from build123d import *

# Parameters (mm, degrees)
SKETCH_R        = 12
SKETCH_R_2      = 8.5
PAD_DEPTH       = 2
SKETCH001_R     = 3
SKETCH001_R_2   = 8.5
PAD001_DEPTH    = 5
SKETCH002_R     = 8.5
PAD002_DEPTH    = 3
SKETCH003_R     = 6.9
PAD003_DEPTH    = 2
PAD004_DEPTH    = 4.5
SKETCH005_R     = 2
PAD005_DEPTH    = 4
FILLET_R        = 3
CHAMFER_SIZE    = 0.4
CHAMFER001_SIZE = 0.4
SKETCH006_R     = 3
POCKET_DEPTH    = 4.001


with BuildPart() as part:
    # Sketch → Pad (new body)
    with BuildSketch(Plane.XY):
        Circle(SKETCH_R)
        Circle(SKETCH_R_2, mode=Mode.SUBTRACT)
    extrude(amount=PAD_DEPTH)

    # Sketch001 (on Face4 of Pad) → Pad001 (join)
    with BuildSketch(Plane.XY.offset(2)):
        with BuildLine():
            ThreePointArc((-1.128054, -11.946861), (12.25, -21.217622), (10.910313, -4.996507))
            ThreePointArc((10.910313, -4.996507), (-6, 10.392305), (-1.128054, -11.946861))
        make_face()
        with Locations((7.75, -13.423394)):
            Circle(SKETCH001_R, mode=Mode.SUBTRACT)
        Circle(SKETCH001_R_2, mode=Mode.SUBTRACT)
    extrude(amount=-PAD001_DEPTH)

    # Sketch002 (on Face6 of Pad001) → Pad002 (join)
    with BuildSketch(Plane(origin=(0, 0, -3), x_dir=(1, 0, 0), z_dir=(0, 0, -1))):
        Circle(SKETCH002_R)
    extrude(amount=-PAD002_DEPTH)

    # Sketch003 (on Face11 of Pad002) → Pad003 (join)
    with BuildSketch(Plane.XY):
        Circle(SKETCH003_R)
    extrude(amount=PAD003_DEPTH)

    # Sketch004 (on Face7 of Pad003) → Pad004 (join)
    with BuildSketch(Plane.XY.offset(2)):
        with BuildLine():
            Line((-0.800254, -10.613919), (5.90795, -22.232869))
            ThreePointArc((-0.800254, -10.613919), (-0.044229, -17.923394), (5.90795, -22.232869))
        make_face()
        with BuildLine():
            Line((16.300254, -16.232869), (9.59205, -4.613919))
            ThreePointArc((16.300254, -16.232869), (15.544229, -8.923394), (9.59205, -4.613919))
        make_face()
    extrude(amount=PAD004_DEPTH)

    # Sketch005 (on Face19 of Pad004) → Pad005 (join)
    with BuildSketch(Plane.XY.offset(-3)):
        with BuildLine():
            Line((-39.5, 16), (17.5, 16))
            Line((17.5, 16), (24.5, 16))
            Line((24.5, 16), (30.5, 16))
            Line((30.5, 16), (30.5, -16))
            Line((24.5, -16), (30.5, -16))
            Line((17.5, -16), (24.5, -16))
            Line((17.5, -16), (16.373288, -16))
            ThreePointArc((-0.873288, -16), (7.75, -22.423394), (16.373288, -16))
            Line((-0.873288, -16), (-39.5, -16))
            Line((-39.5, -16), (-39.5, 16))
        make_face()
        with Locations((-35.5, 5)):
            Circle(SKETCH005_R, mode=Mode.SUBTRACT)
        with Locations((-35.5, -5)):
            Circle(SKETCH005_R, mode=Mode.SUBTRACT)
        with Locations((13.5, 5)):
            Circle(SKETCH005_R, mode=Mode.SUBTRACT)
        with Locations((13.5, -5)):
            Circle(SKETCH005_R, mode=Mode.SUBTRACT)
        with Locations((-35.5, 12)):
            Circle(SKETCH005_R, mode=Mode.SUBTRACT)
        with Locations((-35.5, -12)):
            Circle(SKETCH005_R, mode=Mode.SUBTRACT)
        with Locations((20.5, 12)):
            Circle(SKETCH005_R, mode=Mode.SUBTRACT)
        with Locations((20.5, -12)):
            Circle(SKETCH005_R, mode=Mode.SUBTRACT)
        with Locations((26.5, -12)):
            Circle(SKETCH005_R, mode=Mode.SUBTRACT)
        with Locations((26.5, 12)):
            Circle(SKETCH005_R, mode=Mode.SUBTRACT)
    extrude(amount=-PAD005_DEPTH)

    # Fillet
    fillet_edges = [part.edges().sort_by_distance(p)[0] for p in [
        (-39.5, -16, -5),
        (30.5, -16, -5),
        (30.5, 16, -5),
        (-39.5, 16, -5),
    ]]
    fillet(fillet_edges, radius=FILLET_R)

    # Chamfer
    chamfer_edges = [part.edges().sort_by_distance(p)[0] for p in [
        (-6.9, 0, 2),
    ]]
    chamfer(chamfer_edges, length=CHAMFER_SIZE)

    # Chamfer001
    chamfer001_edges = [part.edges().sort_by_distance(p)[0] for p in [
        (-8.5, 0, 2),
    ]]
    chamfer(chamfer001_edges, length=CHAMFER001_SIZE)

    # Sketch006 (on Face23 of Chamfer001) → Pocket (cut, through all)
    with BuildSketch(Plane.XY.offset(-3)):
        with Locations((7.75, -13.423394)):
            Circle(SKETCH006_R)
    extrude(amount=-POCKET_DEPTH, mode=Mode.SUBTRACT)


solid = part.part
The listing builds one solid part. Answer for the finished solid, in the listing's coordinates (mm). A direction names the side the tool comes from. Coordinates: 2 decimals unless noted, no trailing zeros. Order: outer loops, then holes, each group sorted by start corner. A loop starts at its lowest first (then second) coordinate and runs counter-clockwise, first axis right, second up.
Q1. A cutting plane is placed at D-D, the plane y = 11. Write down the section's boundary in (x, z).
Q2. A cutting plane is placed at C-C, the plane z = -4.5. State how many separate pieces and enclosed holes the cut face has, and give its area (3 significant figures).
Q3. Given P1, Ø4, axis at y = 1, z = 5, coming from the -X side; P2, Ø3, axis at x = 21, z = -5, coming from the -Y side; P3, Ø8, axis at x = 5, y = -11.5, coming from the +Z side; P4, Ø8, axis at x = -4, z = 0.5, coming from the -Y side, each flat-ended and moving along its own axis, determine where each tip first touches the part or whether it passes through.
Q4. A cutting plane is placed at A-A, the plane x = 26.5. Write down the section's boundary in (y, z), and give its area (3 significant figures).
Q5. For a pull along Y with two mould halves and no side action, classify faces 4 (the face through (-18, -16, -5)), 5 (the face through (0, 0, 2)), 6 (the face through (-5, 16, -5)), 7 (the face through (-1, -7, 0)) as pulls with the +Y half, pulls with the -Y half, needs draft (parallel to the pull), parting line crosses it, or undercut.
Q6. A cutting plane is placed at B-B, the plane x = -35.5. Write down the section's boundary in (y, z).
Q7. Which of the six approach directions +Z, -Z, +X, -X, +Y, -Y give full straight-line access (tool end or side, diameter ignored) to faces 1 (the face through (11.9, -6.2, -5)), 2 (the face through (22, -16, -5)), 3 (the face through (-33.653, -5.766, -4.972))?
Q8. Consider line 1 (Y direction, x = -35.5, z = -5.95); line 2 (Y direction, x = 25.5, z = -3.5); line 3 (Y direction, x = 26, z = -4.75). Determine where each line is inside the solid, lowest interval first.
Answers follow:
1. outline: (-39.5, -7) - (-37.23, -7) - (-37.23, -3) - (-39.5, -3) - close; (-33.77, -7) - (18.77, -7) - (18.77, -3) - (4.8, -3) - (4.8, 2) - (-4.8, 2) - (-4.8, -3) - (-33.77, -3) - close; (22.23, -7) - (24.77, -7) - (24.77, -3) - (22.23, -3) - close; (28.23, -7) - (30.5, -7) - (30.5, -3) - (28.23, -3) - close
2. separate pieces: 1
2. enclosed holes: 11
2. area: 2,160 mm2
3. P1: passes through
3. P2: stops at y = -16
3. P3: stops at z = 2
3. P4: stops at y = -18
4. outline: (-16, -7) - (-14, -7) - (-14, -3) - (-16, -3) - close; (-10, -7) - (10, -7) - (10, -3) - (-10, -3) - close; (14, -7) - (16, -7) - (16, -3) - (14, -3) - close
4. area: 96.0 mm2
5. face 4: pulls with the -Y half
5. face 5: needs draft
5. face 6: pulls with the +Y half
5. face 7: undercut
6. outline: (-16, -7) - (-14, -7) - (-14, -3) - (-16, -3) - close; (-10, -7) - (-7, -7) - (-7, -3) - (-10, -3) - close; (-3, -7) - (3, -7) - (3, -3) - (-3, -3) - close; (7, -7) - (10, -7) - (10, -3) - (7, -3) - close; (14, -7) - (16, -7) - (16, -3) - (14, -3) - close
7. face 1: -Z
7. face 2: +Z, -Z, +X, -Y
7. face 3: +Z, -Z
8. line 1: y = -16 to -14, -10 to -7, -3 to 3, 7 to 10, 14 to 16
8. line 2: y = -16 to -13.73, -10.27 to 10.27, 13.73 to 16
8. line 3: y = -16 to -13.94, -10.06 to 10.06, 13.94 to 16
